Input: part model. Units: mm. Frame: model coordinates. Face numbers are marked on the shaded views. A direction names the side the tool comes from. Give positions to 0.01 mm unless a question says otherwise; leave off trailing zeros. Loops run counter-clockwise (first coordinate to the right, second up) from the corner with the lowest first, then second, coordinate; pieces in that order, holes last. Notation, with made-up numbers: (-10, 40) - (0, 40) arc R27 cw to (0, 71) - close; hole circle Ø5 at (14, 82.5). An arc over 180 degrees is marked (long way). Answer as a JSON object with one key per item and string values. Group by question number.
(1) Section query B-B (z = -4.75). Count the separate pieces of the cut face and the enclosed holes in it, plus the area to 3 significant figures.
(2) Mould query, pull axis Z, two halves, no side actions, for the marked faces 1, 2 and 3. Classes: +Z half, -Z half, draft (parallel to the pull), parting line (faces both ways), or undercut.
(3) Access query for the marked faces 4 and 5. Directions: +Z, -Z, +X, -X, +Y, -Y. A direction counts if a zero-diameter tool reaches every point of the face in a straight line with its end or side. Return the directions, or none.
(4) Section query D-D (z = -11.75). Return loops of the section in (x, y), plus the area to 3 significant figures.
(5) Material intervals for L1, parallel to Z at x = 20, y = 2.25; L2, parallel to X at y = 7, z = 1; L3, parallel to X at y = 1, z = -8, sorted ascending.
(6) Section query C-C (y = 7.25). Return loops of the section in (x, z), plus the area to 3 significant figures.
(7) Section query A-A (x = -8). Return loops of the section in (y, z), plus the area to 3 significant figures.
(8) Pin query (flat end, axial travel): P1, Ø17.5, axis at x = 1, z = -1, coming from the +Y side. Return the tip coordinate at first contact, or that it passes through.
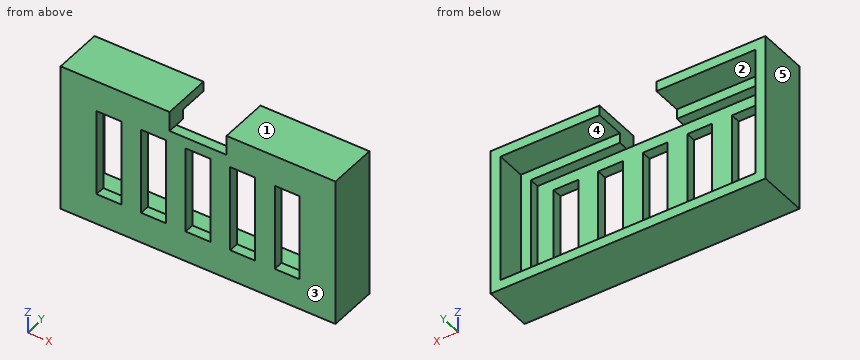
```python
from build123d import *

# Parameters (mm, degrees)
BOSS_EXTRUDE1_DEPTH = 4
BOSS_EXTRUDE3_DEPTH = 10
BOSS_EXTRUDE4_DEPTH = 2
SKETCH2_W           = 5
SKETCH2_H           = 17.5
CUT_EXTRUDE2_DEPTH  = 2


with BuildPart() as part:
    # Sketch1 → Boss-Extrude1 (new body)
    with BuildSketch(Plane(origin=(0, 0, 0), x_dir=(1, 0, 0), z_dir=(0, 1, 0))):
        Polygon((5.75, -11), (5.75, -13), (25.75, -13), (25.75, 13), (-25.75, 13), (-25.75, -13), (-5.75, -13), (-5.75, -11), (-23.75, -11), (-23.75, 11), (23.75, 11), (23.75, -11), align=None)
    extrude(amount=BOSS_EXTRUDE1_DEPTH)

    # Sketch1_4 → Boss-Extrude3 (add)
    with BuildSketch(Plane(origin=(0, 0, 0), x_dir=(1, 0, 0), z_dir=(0, 1, 0))):
        Polygon((27.75, -15), (27.75, 15), (-27.75, 15), (-27.75, -15), (-5.75, -15), (-5.75, -13), (-25.75, -13), (-25.75, 13), (25.75, 13), (25.75, -13), (5.75, -13), (5.75, -15), align=None)
    extrude(amount=BOSS_EXTRUDE3_DEPTH)

    # Sketch1_6 → Boss-Extrude4 (add)
    with BuildSketch(Plane(origin=(0, 0, 0), x_dir=(1, 0, 0), z_dir=(0, 1, 0))):
        Polygon((-5.75, -11), (-23.75, -11), (-23.75, 11), (23.75, 11), (23.75, -11), (5.75, -11), align=None)
    extrude(amount=BOSS_EXTRUDE4_DEPTH)

    # Sketch2 → Cut-Extrude2 (cut)
    with BuildSketch(Plane(origin=(0, 2, 0), x_dir=(1, 0, 0), z_dir=(0, 1, 0))):
        with Locations((9, 0)):
            Rectangle(SKETCH2_W, SKETCH2_H)
        Rectangle(SKETCH2_W, SKETCH2_H)
        with Locations((18, 0)):
            Rectangle(SKETCH2_W, SKETCH2_H)
        with Locations((-9, 0)):
            Rectangle(SKETCH2_W, SKETCH2_H)
        with Locations((-18, 0)):
            Rectangle(SKETCH2_W, SKETCH2_H)
    extrude(amount=-CUT_EXTRUDE2_DEPTH, mode=Mode.SUBTRACT)


solid = part.part
```
Recorded:
{
 "1": {"separate pieces": "6", "enclosed holes": "0", "area": "101 mm^2"},
 "2": {"face 1": "+Z half", "face 2": "undercut", "face 3": "draft"},
 "3": {"face 4": "+Y", "face 5": "+Z, -Z, -X, +Y, -Y"},
 "4": {"outline": "(-27.75, 0) - (27.75, 0) - (27.75, 10) - (25.75, 10) - (25.75, 4) - (-25.75, 4) - (-25.75, 10) - (-27.75, 10) - close", "area": "246 mm^2"},
 "5": {"L1": "z = -15 to -11, 11 to 15", "L2": "x = -27.75 to -25.75, 25.75 to 27.75", "L3": "x = -27.75 to -20.5, -15.5 to -11.5, -6.5 to -2.5, 2.5 to 6.5, 11.5 to 15.5, 20.5 to 27.75"},
 "6": {"outline": "(-27.75, -15) - (27.75, -15) - (27.75, 15) - (5.75, 15) - (5.75, 13) - (25.75, 13) - (25.75, -13) - (-25.75, -13) - (-25.75, 13) - (-5.75, 13) - (-5.75, 15) - (-27.75, 15) - close", "area": "303 mm^2"},
 "7": {"outline": "(0, -15) - (10, -15) - (10, -13) - (4, -13) - (4, -11) - (2, -11) - (2, -8.75) - (0, -8.75) - close; (0, 8.75) - (2, 8.75) - (2, 11) - (4, 11) - (4, 13) - (10, 13) - (10, 15) - (0, 15) - close", "area": "65.0 mm^2"},
 "8": {"P1": "stops at y = 2"}
}
